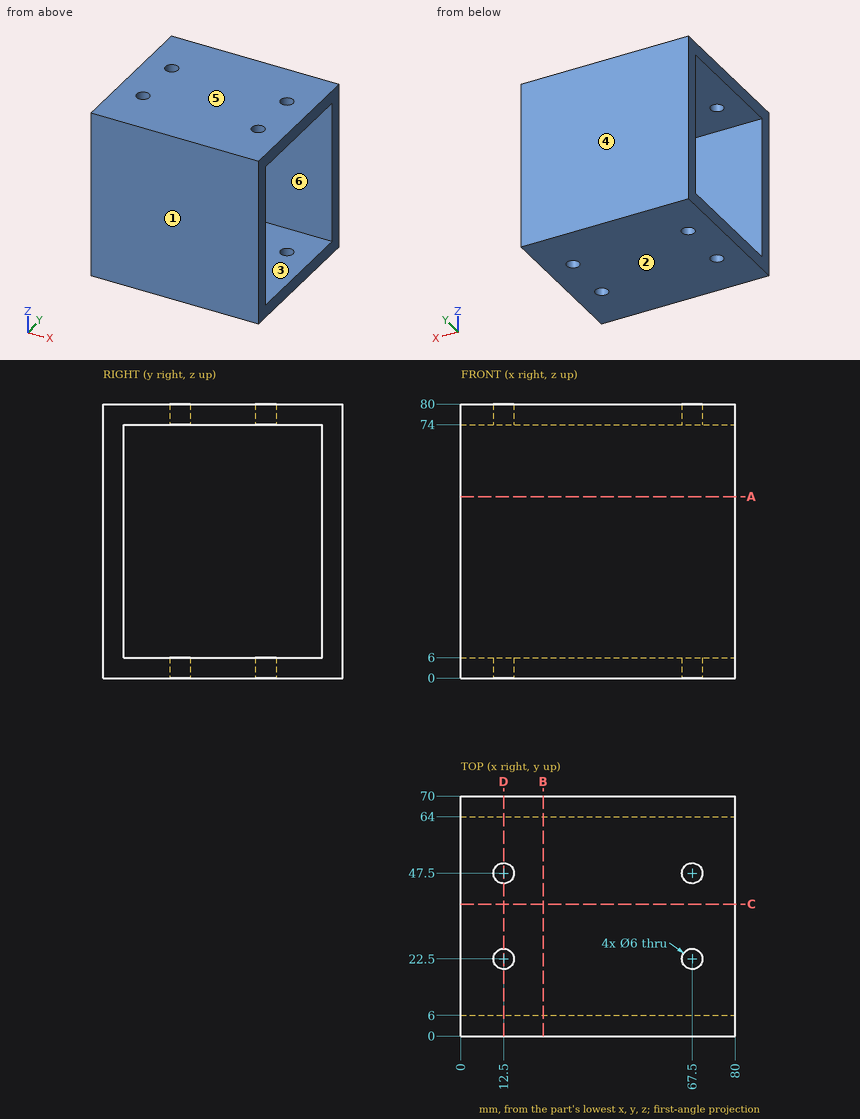
Could you check a few things on this drawing? It's one solid part, dimensions in mm from its lowest x, y, z. A direction names the side the tool comes from. Coordinates: 2 decimals unless noted, no trailing zeros. Loops run counter-clockwise (first coordinate to the right, second up) from the corner with the lowest first, then second, coordinate; pieces in that order, holes last.
1. Imagine slicing it at B-B (x = 24). Please give me the cut outline in (y, z), and give its area (3 significant figures).
2. We'd pull the mould along Y, two halves only. Please class the marked faces 1, 2, 3 and 4: released by +Y, released by -Y, zero draft, split by the parting line, or undercut.
3. Imagine slicing it at C-C (y = 38.5). Please give me the cut outline in (x, z).
4. I need wall thicknesses on L1, parallel to Y at x = 67.5, z = 1.6; L2, parallel to Z at x = 44, y = 29; L3, parallel to Y at x = 22, z = 65.5. Which ranges of each line are inside material? Lowest first, please.
5. For P1, Ø7, axis at x = 67.5, y = 22.5, coming from the -Z side, with a flat end and sliding along its axis, tell me the tip position at first contact or that it passes through.
6. For the marked faces 5 and 6, which set-ups out of +Z, -Z, +X, -X, +Y, -Y let a thin tool reach every point of the face, with its end or its side?
7. Imagine slicing it at A-A (z = 53). Please give me the cut outline in (x, y), and give its area (3 significant figures).
8. Imagine slicing it at D-D (x = 12.5). Please give me the cut outline in (y, z).
Computed values:
1. outline: (0, 0) - (70, 0) - (70, 80) - (0, 80) - close; hole (6, 6) - (64, 6) - (64, 74) - (6, 74) - close
1. area: 1,660 mm2
2. face 1: released by -Y
2. face 2: zero draft
2. face 3: undercut
2. face 4: released by +Y
3. outline: (0, 0) - (80, 0) - (80, 6) - (0, 6) - close; (0, 74) - (80, 74) - (80, 80) - (0, 80) - close
4. L1: y = 0 to 19.5, 25.5 to 44.5, 50.5 to 70
4. L2: z = 0 to 6, 74 to 80
4. L3: y = 0 to 6, 64 to 70
5. P1: stops at z = 0
6. face 5: +Z, +X, -X, +Y, -Y
6. face 6: +X, -X
7. outline: (0, 0) - (80, 0) - (80, 6) - (0, 6) - close; (0, 64) - (80, 64) - (80, 70) - (0, 70) - close
7. area: 960 mm2
8. outline: (0, 0) - (19.5, 0) - (19.5, 6) - (6, 6) - (6, 74) - (19.5, 74) - (19.5, 80) - (0, 80) - close; (25.5, 0) - (44.5, 0) - (44.5, 6) - (25.5, 6) - close; (25.5, 74) - (44.5, 74) - (44.5, 80) - (25.5, 80) - close; (50.5, 0) - (70, 0) - (70, 80) - (50.5, 80) - (50.5, 74) - (64, 74) - (64, 6) - (50.5, 6) - close
